Autodesk Inventor part; units mm, degrees
ref_plane "YZ Plane" through (0, 0, 0) normal (1, 0, 0) x (0, 1, 0)
ref_plane "XZ Plane" through (0, 0, 0) normal (0, 1, 0) x (-1, 0, 0)
ref_plane "XY Plane" through (0, 0, 0) normal (0, 0, 1) x (1, 0, 0)
sketch "Sketch1" plane through (0, 0, 0) normal (0, 1, 0) x (-1, 0, 0)
  line L0 (-266.0977, 629.1478) -> (143.9023, 629.1478)
  line L1 (143.9023, 629.1478) -> (143.9023, -80.8522)
  line L2 (143.9023, -80.8522) -> (-266.0977, -80.8522)
  line L3 (-266.0977, -80.8522) -> (-266.0977, 629.1478)
  circle A0 centre (-61.0977, 579.1478) radius 25
  circle A1 centre (-61.0977, -30.8522) radius 25
  point P0 (0, 0)
  dimension "d0" = 710
  dimension "d1" = 410
  dimension "d4" = 50
  dimension "d5" = 50
extrude "Extrusion1" add sketch "Sketch1" along normal blind 3
sketch "Sketch2" plane through (266.0977, 0, 629.1478) normal (1, 0, 0) x (0, 0, -1)
  line L0 (710, 3) -> (0, 3)
  line L1 (710, 3) -> (0, 3)
  line L2 (0, 3) -> (0, 0)
  line L3 (0, 0) -> (710, 0)
  line L4 (710, 0) -> (710, 3)
  line L5 (355, 0) -> (525, 0)
  line L6 (710, 0) -> (0, 0)
  line L7 (355, 3) -> (185, 3)
  line L8 (185, 3) -> (525, 3)
  line L9 (525, 3) -> (525, 0)
  line L10 (525, 0) -> (185, 0)
  line L11 (185, 0) -> (185, 3)
  point P0 (629.1478, 0)
  dimension "d8" = 170
  dimension "d9" = 170
extrude "Extrusion2" add sketch "Sketch2" along normal blind 2000 contours L9 L3 L11 L0
sketch "Sketch3" plane through (0, 3, 0) normal (0, 1, 0) x (1, 0, 0)
  line L0 (2266.0977, -104.1478) -> (2266.0977, -444.1478)
  line L1 (266.0977, -104.1478) -> (2266.0977, -104.1478)
  line L2 (2266.0977, -444.1478) -> (2236.0977, -444.1478)
  line L3 (2236.0977, -444.1478) -> (2236.0977, -104.1478)
  line L4 (2236.0977, -104.1478) -> (2266.0977, -104.1478)
  line L5 (2266.0977, -104.1478) -> (2266.0977, -444.1478)
  point P0 (0, 0)
  dimension "d12" = 340
  dimension "d13" = 30
extrude "Extrusion3" add sketch "Sketch3" along normal blind 200
sketch "Sketch4" plane through (266.0977, 0, 444.1478) normal (0, 0, 1) x (1, 0, 0)
  line L0 (1970, 3) -> (1970, 203)
  line L1 (1970, 203) -> (1970, 2.607)
  line L2 (0, 0) -> (2000, 0)
  line L3 (1970, 203) -> (1758.8495, 2.607)
  line L4 (1758.8495, 2.607) -> (1970, 2.607)
  line L5 (1970, 203) -> (1970, 2.607)
  point P0 (-266.0977, 0)
extrude "Extrusion4" add sketch "Sketch4" against normal blind 30
sketch "Sketch5" plane through (0, 3, 0) normal (0, 1, 0) x (1, 0, 0)
  line L0 (266.0977, 80.8522) -> (-143.9023, 80.8522)
  line L1 (-143.9023, 80.8522) -> (2266.0977, 80.8522)
  line L2 (-143.9023, 80.8522) -> (-143.9023, -629.1478)
  line L3 (-143.9023, 80.8522) -> (-143.9023, -629.1478)
  point P0 (0, 0)
  dimension "d18" = 2410
  dimension "d19" = 710
properties part number "soporte"
Input: part model. Units: mm. Frame: model coordinates. A direction names the side the tool comes from. Give positions to 0.01 mm unless a question says otherwise; leave off trailing zeros. Order: outer loops, then holes, each group sorted by start corner. A loop starts at its lowest first (then second) coordinate and runs counter-clockwise, first axis right, second up.
Q1. Section C-C on x = 1757.5. Output: boundary loops of the cut face in (y, z), and give its area (3 significant figures).
Checked values:
outline: (0, 104.15) - (3, 104.15) - (3, 444.15) - (0, 444.15) - close
area: 1,020 mm2
Q2. Contact query for flat-ended pins moving along their axis: pin 1 Ø6 at (x, z) = (204, 27) entering from +Y; pin 2 Ø0.9 at (y, z) = (1, -23.5) entering from +X. Output: stop coordinate, or through.
Checked values:
pin 1: stops at y = 3
pin 2: stops at x = 266.1
Q3. Section B-B on y = 31.5. Output: boundary loops of the cut face in (x, z), and give its area (3 significant figures).
Checked values:
outline: (2055.39, 414.15) - (2236.1, 414.15) - (2236.1, 104.15) - (2266.1, 104.15) - (2266.1, 444.15) - (2055.39, 444.15) - close
area: 15,600 mm2
Q4. Section D-D on z = 31. Output: boundary loops of the cut face in (x, y), and give its area (3 significant figures).
Checked values:
outline: (-143.9, 0) - (266.1, 0) - (266.1, 3) - (-143.9, 3) - close
area: 1,230 mm2
Q5. Set-up query: faces 1 (the flat face through (2132.205, 104.4, 429.358)), 2 (the flat face through (2236.098, 102, 261)). Return all of +Z, -Z, +X, -X, +Y, -Y with unobstructed straight access to the full face (end or side cutting, diameter ignored); none if empty.
Checked values:
face 1: +Z, -Z, -X, +Y
face 2: -Z, -X, +Y
Q6. Ray query, probe 1 along X at (y, z) = (41, 308); probe 2 along Y at (x, z) = (1650, 428.5); probe 3 along X at (y, z) = (59, 425.5). Return the intervals inside material, ascending.
Checked values:
probe 1: x = 2236.1 to 2266.1
probe 2: y = 0 to 3
probe 3: x = 2084.37 to 2266.1
Q7. Section A-A on z = 317.5. Output: boundary loops of the cut face in (x, y).
Checked values:
outline: (-143.9, 0) - (2266.1, 0) - (2266.1, 203) - (2236.1, 203) - (2236.1, 3) - (-143.9, 3) - close
Q8. Draft query along Z for faces 3 (the flat face through (2176, 60, 414.148)), 4 (the cylindrical face through (37.25, 1.48, -38.36)), 5 (the flat face through (1063, 3, 279)), 6 (the cylindrical face through (47.658, 1.479, 558.068)). Return one class per face: +Z half, -Z half, draft (parallel to the pull), parting line (faces both ways), or undercut.
Checked values:
face 3: -Z half
face 4: undercut
face 5: draft
face 6: undercut
